Check sheet for the modelled part. Datum: model origin and axes. Units: mm. A direction names the side the tool comes from. Give positions to 0.01 mm unless a question says otherwise; leave off trailing zeros. Order: outer loops, then holes, each group sorted by start corner. A loop starts at its lowest first (then second) coordinate and runs counter-clockwise, first axis right, second up. Notation, with made-up numbers: (1, 29) -> (29, 29) arc R27 cw to (29, 47) -> close; hole circle Ø5 at (49, 5). An arc over 180 degrees is marked (long way). Answer in a Markdown table with one row per item. Add a question column.
(1) Set-up check for faces 1 (the face through (-25, 0, -1)), 2 (the face through (-8.8, -2, 7)), 3 (the face through (27, 13, 0)): record each of +Z, -Z, +X, -X, +Y, -Y from which the full face is reachable in a straight line by a thin tool's end or side.
(2) Cross-section at B-B (y = 20). Record the cut outline in (x, z), then the cut area to 3 significant figures.
(3) Cross-section at D-D (y = -6.5). Record the cut outline in (x, z), then the cut area to 3 significant figures.
(4) Go/stop test with flat-tipped pins: pin 1 (3 mm diameter, centred on x = -8, z = 3, fed in from -Y); pin 2 (4 mm diameter, centred on y = -15, z = -0.5, fed in from +X); pin 3 (1 mm diameter, centred on y = 9.5, z = -1, fed in from -X); pin 4 (5.5 mm diameter, centred on x = 27, z = 1.5, fed in from -Y). Record where each tip stops, or that it passes through.
(5) Release check for a two-part mould opening along Y. For faces 4 (the face through (-20, -10.2, 7)), 5 (the face through (0, 25, -1)), 6 (the face through (-21.537, 20.202, -1.014)), 7 (the face through (-20, -2, 13.5)) record: released by +Y, released by -Y, zero draft, split by the parting line, or undercut.
(6) Cross-section at C-C (x = -20). Record the cut outline in (y, z), then the cut area to 3 significant figures.
(7) Thickness scan on L1, parallel to X at y = 20, z = -0.7; L2, parallel to Y at x = 27, z = 4.5. Record the ranges inside material, lowest first. Write a range as [from, to].
(8) Cross-section at A-A (z = 7). Record the cut outline in (x, y).
Autodesk Inventor part; units mm, degrees
ref_plane "YZ Plane" through (0, 0, 0) normal (1, 0, 0) x (0, 1, 0)
ref_plane "XZ Plane" through (0, 0, 0) normal (0, 1, 0) x (-1, 0, 0)
ref_plane "XY Plane" through (0, 0, 0) normal (0, 0, 1) x (1, 0, 0)
sketch "Platine" plane through (0, 0, 0) normal (0, 0, 1) x (1, 0, 0)
  line L0 (-25, -25) -> (25, -25)
  line L1 (25, -25) -> (25, 25)
  line L2 (25, 25) -> (-25, 25)
  line L3 (-25, 25) -> (-25, -25)
  line L4 (-25, -25) -> (25, 25)
  line L5 (25, -25) -> (-25, 25)
  line L6 (-30.8, -10.2) -> (-8.8, -10.2)
  line L7 (-8.8, -10.2) -> (-8.8, 5.8)
  line L8 (-8.8, 5.8) -> (-30.8, 5.8)
  line L9 (-30.8, 5.8) -> (-30.8, -10.2)
  line L10 (33.4, -11.2) -> (19.4, -11.2)
  line L11 (19.4, -11.2) -> (19.4, -1.04)
  line L12 (19.4, -1.04) -> (33.4, -1.04)
  line L13 (33.4, -1.04) -> (33.4, -11.2)
  line L14 (14.5, 8) -> (28.5, 8)
  line L15 (28.5, 8) -> (28.5, 18)
  line L16 (28.5, 18) -> (14.5, 18)
  line L17 (14.5, 18) -> (14.5, 8)
  circle A0 centre (-20, 20) radius 1.5
  circle A1 centre (20, -20) radius 1.5
  point P0 (0, 0)
  point P1 (0, 0)
  dimension "d0" = 50
  dimension "d1" = 50
  dimension "d2" = 22
  dimension "d3" = 16
  dimension "d4" = 14.8
  dimension "d5" = 5.8
  dimension "d6" = 14
  dimension "d7" = 10.16
  dimension "d8" = 13.8
  dimension "d9" = 44.4
  dimension "d10" = 10
  dimension "d11" = 14
  dimension "d12" = 33
  dimension "d13" = 10.5
  dimension "d14" = 3
  dimension "d15" = 5
  dimension "d16" = 5
  dimension "d17" = 5
  dimension "d18" = 5
  dimension "d19" = 18
  dimension "d20" = 33.4
extrude "Platinengeometrie" add sketch "Platine" against normal blind 2 contours L4 L6 L7 L5 A1 L0 | L3 L6 L4 | L5 A1 L4 L17 L14 L1 L12 L11 L10 | L3 L8 L7 L4 L6 | L4 L7 L6 | L10 L11 L12 L1 | A1 L5 | L5 A1 | L3 L5 A0 L4 L7 L8 | L2 L4 L16 L17 L5 A0 | L14 L17 L4 L16 L1 | L1 L16 L4 | A0 L5 | L5 A0 | L17 L16 L4
sketch "Platine2" plane through (0, 0, 0) normal (0, 0, 1) x (1, 0, 0)
  line L0 (-25, -25) -> (25, -25)
  line L1 (25, -25) -> (25, 25)
  line L2 (25, 25) -> (-25, 25)
  line L3 (-25, 25) -> (-25, -25)
  line L4 (-25, -25) -> (25, 25)
  line L5 (25, -25) -> (-25, 25)
  line L6 (-30.8, -10.2) -> (-8.8, -10.2)
  line L7 (-8.8, -10.2) -> (-8.8, 5.8)
  line L8 (-8.8, 5.8) -> (-30.8, 5.8)
  line L9 (-30.8, 5.8) -> (-30.8, -10.2)
  line L10 (33.4, -11.2) -> (19.4, -11.2)
  line L11 (19.4, -11.2) -> (19.4, -1.04)
  line L12 (19.4, -1.04) -> (33.4, -1.04)
  line L13 (33.4, -1.04) -> (33.4, -11.2)
  line L14 (14.5, 8) -> (28.5, 8)
  line L15 (28.5, 8) -> (28.5, 18)
  line L16 (28.5, 18) -> (14.5, 18)
  line L17 (14.5, 18) -> (14.5, 8)
  circle A0 centre (-20, 20) radius 1.5
  circle A1 centre (20, -20) radius 1.5
  point P0 (0, 0)
  point P1 (0, 0)
  point P2 (0, 0)
  dimension "d23" = 50
  dimension "d24" = 50
  dimension "d25" = 22
  dimension "d26" = 16
  dimension "d27" = 14.8
  dimension "d28" = 5.8
  dimension "d29" = 14
  dimension "d30" = 10.16
  dimension "d31" = 13.8
  dimension "d32" = 44.4
  dimension "d33" = 10
  dimension "d34" = 14
  dimension "d35" = 33
  dimension "d36" = 10.5
  dimension "d37" = 3
  dimension "d38" = 5
  dimension "d39" = 5
  dimension "d40" = 5
  dimension "d41" = 5
  dimension "d42" = 18
  dimension "d43" = 33.4
extrude "MEBP 8-8G" add sketch "Platine2" along normal blind 13.5 contours L6 L9 L8 L3 | L3 L8 L7 L4 L6 | L4 L7 L6
sketch "Platine3" plane through (0, 0, 0) normal (0, 0, 1) x (1, 0, 0)
  line L0 (-25, -25) -> (25, -25)
  line L1 (25, -25) -> (25, 25)
  line L2 (25, 25) -> (-25, 25)
  line L3 (-25, 25) -> (-25, -25)
  line L4 (-25, -25) -> (25, 25)
  line L5 (25, -25) -> (-25, 25)
  line L6 (-30.8, -10.2) -> (-8.8, -10.2)
  line L7 (-8.8, -10.2) -> (-8.8, 5.8)
  line L8 (-8.8, 5.8) -> (-30.8, 5.8)
  line L9 (-30.8, 5.8) -> (-30.8, -10.2)
  line L10 (33.4, -11.2) -> (19.4, -11.2)
  line L11 (19.4, -11.2) -> (19.4, -1.04)
  line L12 (19.4, -1.04) -> (33.4, -1.04)
  line L13 (33.4, -1.04) -> (33.4, -11.2)
  line L14 (14.5, 8) -> (28.5, 8)
  line L15 (28.5, 8) -> (28.5, 18)
  line L16 (28.5, 18) -> (14.5, 18)
  line L17 (14.5, 18) -> (14.5, 8)
  circle A0 centre (-20, 20) radius 1.5
  circle A1 centre (20, -20) radius 1.5
  point P0 (0, 0)
  point P1 (0, 0)
  point P2 (0, 0)
  dimension "d46" = 50
  dimension "d47" = 50
  dimension "d48" = 22
  dimension "d49" = 16
  dimension "d50" = 14.8
  dimension "d51" = 5.8
  dimension "d52" = 14
  dimension "d53" = 10.16
  dimension "d54" = 13.8
  dimension "d55" = 44.4
  dimension "d56" = 10
  dimension "d57" = 14
  dimension "d58" = 33
  dimension "d59" = 10.5
  dimension "d60" = 3
  dimension "d61" = 5
  dimension "d62" = 5
  dimension "d63" = 5
  dimension "d64" = 5
  dimension "d65" = 18
  dimension "d66" = 33.4
extrude "PSS 254/4W" add sketch "Platine3" along normal blind 5 contours L10 L11 L12 L1 | L1 L12 L13 L10
sketch "Sketch4" plane through (0, 0, 0) normal (0, 0, 1) x (1, 0, 0)
  line L0 (-25, -25) -> (25, -25)
  line L1 (25, -25) -> (25, 25)
  line L2 (25, 25) -> (-25, 25)
  line L3 (-25, 25) -> (-25, -25)
  line L4 (-25, -25) -> (25, 25)
  line L5 (25, -25) -> (-25, 25)
  line L6 (-30.8, -10.2) -> (-8.8, -10.2)
  line L7 (-8.8, -10.2) -> (-8.8, 5.8)
  line L8 (-8.8, 5.8) -> (-30.8, 5.8)
  line L9 (-30.8, 5.8) -> (-30.8, -10.2)
  line L10 (33.4, -11.2) -> (19.4, -11.2)
  line L11 (19.4, -11.2) -> (19.4, -1.04)
  line L12 (19.4, -1.04) -> (33.4, -1.04)
  line L13 (33.4, -1.04) -> (33.4, -11.2)
  line L14 (14.5, 8) -> (28.5, 8)
  line L15 (28.5, 8) -> (28.5, 18)
  line L16 (28.5, 18) -> (14.5, 18)
  line L17 (14.5, 18) -> (14.5, 8)
  circle A0 centre (-20, 20) radius 1.5
  circle A1 centre (20, -20) radius 1.5
  point P0 (0, 0)
  point P1 (0, 0)
  point P2 (0, 0)
  dimension "d69" = 50
  dimension "d70" = 50
  dimension "d71" = 22
  dimension "d72" = 16
  dimension "d73" = 14.8
  dimension "d74" = 5.8
  dimension "d75" = 14
  dimension "d76" = 10.16
  dimension "d77" = 13.8
  dimension "d78" = 44.4
  dimension "d79" = 10
  dimension "d80" = 14
  dimension "d81" = 33
  dimension "d82" = 10.5
  dimension "d83" = 3
  dimension "d84" = 5
  dimension "d85" = 5
  dimension "d86" = 5
  dimension "d87" = 5
  dimension "d88" = 18
  dimension "d89" = 33.4
extrude "HEBG9 25" add sketch "Sketch4" along normal blind 10 contours L14 L17 L4 L16 L1 | L1 L16 L15 L14 | L17 L16 L4
sketch "Sketch5" plane through (0, 0, 0) normal (0, 0, 1) x (1, 0, 0)
  line L0 (-25, -25) -> (25, -25)
  line L1 (25, -25) -> (25, 25)
  line L2 (25, 25) -> (-25, 25)
  line L3 (-25, 25) -> (-25, -25)
  line L4 (-25, -25) -> (25, 25)
  line L5 (25, -25) -> (-25, 25)
  line L6 (-30.8, -10.2) -> (-8.8, -10.2)
  line L7 (-8.8, -10.2) -> (-8.8, 5.8)
  line L8 (-8.8, 5.8) -> (-30.8, 5.8)
  line L9 (-30.8, 5.8) -> (-30.8, -10.2)
  line L10 (33.4, -11.2) -> (19.4, -11.2)
  line L11 (19.4, -11.2) -> (19.4, -1.04)
  line L12 (19.4, -1.04) -> (33.4, -1.04)
  line L13 (33.4, -1.04) -> (33.4, -11.2)
  line L14 (14.5, 8) -> (28.5, 8)
  line L15 (28.5, 8) -> (28.5, 18)
  line L16 (28.5, 18) -> (14.5, 18)
  line L17 (14.5, 18) -> (14.5, 8)
  circle A0 centre (-20, 20) radius 1.5
  circle A1 centre (20, -20) radius 1.5
  point P0 (0, 0)
  point P1 (0, 0)
  point P2 (0, 0)
  dimension "d92" = 50
  dimension "d93" = 50
  dimension "d94" = 22
  dimension "d95" = 16
  dimension "d96" = 14.8
  dimension "d97" = 5.8
  dimension "d98" = 14
  dimension "d99" = 10.16
  dimension "d100" = 13.8
  dimension "d101" = 44.4
  dimension "d102" = 10
  dimension "d103" = 14
  dimension "d104" = 33
  dimension "d105" = 10.5
  dimension "d106" = 3
  dimension "d107" = 5
  dimension "d108" = 5
  dimension "d109" = 5
  dimension "d110" = 5
  dimension "d111" = 18
  dimension "d112" = 33.4
hole "Hole1" at (-20, 20, 0) at (20, -20, 0) direction (0, 0, -1) diameter 3.1 end through all
properties part number "PCB-Model"
Answer below:
| question | item | result |
|---|---|---|
| 1 | face 1 | -Z, -X, +Y, -Y |
| 1 | face 2 | +Z, +Y, -Y |
| 1 | face 3 | -Z, +X, +Y, -Y |
| 2 | outline | (-25, -2) -> (-21.55, -2) -> (-21.55, 0) -> (-25, 0) -> close; (-18.45, -2) -> (25, -2) -> (25, 0) -> (-18.45, 0) -> close |
| 2 | area | 93.8 mm² |
| 3 | outline | (-30.8, 0) -> (-25, 0) -> (-25, -2) -> (25, -2) -> (25, 0) -> (33.4, 0) -> (33.4, 5) -> (19.4, 5) -> (19.4, 0) -> (-8.8, 0) -> (-8.8, 13.5) -> (-30.8, 13.5) -> close |
| 3 | area | 467 mm² |
| 4 | pin 1 | stops at y = -10.2 |
| 4 | pin 2 | stops at x = 25 |
| 4 | pin 3 | stops at x = -25 |
| 4 | pin 4 | stops at y = -25 |
| 5 | face 4 | released by -Y |
| 5 | face 5 | released by +Y |
| 5 | face 6 | undercut |
| 5 | face 7 | zero draft |
| 6 | outline | (-25, -2) -> (18.45, -2) -> (18.45, 0) -> (5.8, 0) -> (5.8, 13.5) -> (-10.2, 13.5) -> (-10.2, 0) -> (-25, 0) -> close; (21.55, -2) -> (25, -2) -> (25, 0) -> (21.55, 0) -> close |
| 6 | area | 310 mm² |
| 7 | L1 | x = [-25, -21.55], [-18.45, 25] |
| 7 | L2 | y = [-11.2, -1.04], [8, 18] |
| 8 | outline | (-30.8, -10.2) -> (-8.8, -10.2) -> (-8.8, 5.8) -> (-30.8, 5.8) -> close; (14.5, 8) -> (28.5, 8) -> (28.5, 18) -> (14.5, 18) -> close |
